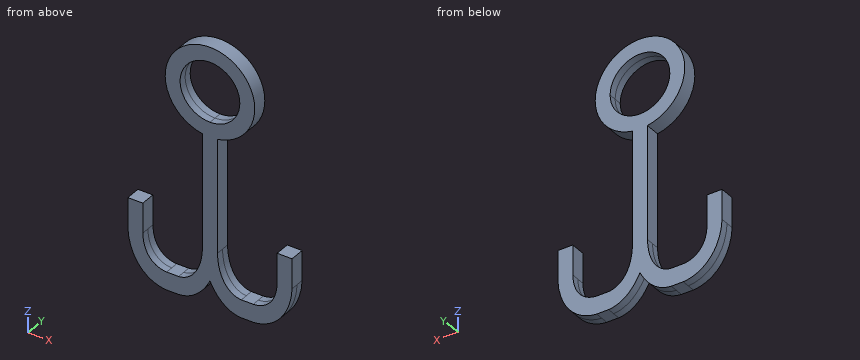
from build123d import *

# Parameters (mm, degrees)
F0_W     = 25.4
F0_H     = 38.1
F0_W_2   = 31.75
F0_H_2   = 63.5
F1_DEPTH = 15.875


with BuildPart() as f1:
    # F0 (on Front) → F1 (new body, symmetric)
    with BuildSketch(Plane.XZ):
        with BuildLine():
            Line((-15.875, -103.8391655019), (-15.875, -345.1981674205))
            Line((-15.875, -345.1981674205), (0, -345.1981674205))
            Line((0, -345.1981674205), (0, -105.1713989452))
            ThreePointArc((0, -105.1713989452), (-7.9654012916, -104.8377562407), (-15.875, -103.8391655019))
        make_face()
        with BuildLine():
            add(Edge.make_bspline(
                [(0, -409.482145582), (-10.3991862171, -388.0156164118), (-15.7271620535, -363.9765002128), (-15.875, -345.1981674205)],
                knots=[81.5477604067, 81.5477604067, 81.5477604067, 81.5477604067, 143.8364349915, 143.8364349915, 143.8364349915, 143.8364349915], degree=3))
            add(Edge.make_bspline(
                [(-66.675, -424.8878848455), (-44.6960218251, -423.8382875919), (-17.5926852971, -402.3276865482), (-15.875, -345.1981674205)],
                knots=[0, 0, 0, 0, 94.5044499655, 94.5044499655, 94.5044499655, 94.5044499655], degree=3))
            Line((-66.675, -424.8878848455), (-66.675, -462.9878848455))
            add(Edge.make_bspline(
                [(-66.675, -462.9878848455), (-35.9209941881, -461.2803468487), (-13.6145190391, -437.5859283193), (0, -409.482145582)],
                knots=[0, 0, 0, 0, 81.5477604067, 81.5477604067, 81.5477604067, 81.5477604067], degree=3))
        make_face()
        with BuildLine():
            Line((0, -345.1981674205), (-15.875, -345.1981674205))
            add(Edge.make_bspline(
                [(0, -409.482145582), (-10.3991862171, -388.0156164118), (-15.7271620535, -363.9765002128), (-15.875, -345.1981674205)],
                knots=[81.5477604067, 81.5477604067, 81.5477604067, 81.5477604067, 143.8364349915, 143.8364349915, 143.8364349915, 143.8364349915], degree=3))
            add(Edge.make_bspline(
                [(0, -409.482145582), (10.3991862171, -388.0156164118), (15.7271620535, -363.9765002128), (15.875, -345.1981674205)],
                knots=[81.5477604067, 81.5477604067, 81.5477604067, 81.5477604067, 143.8364349915, 143.8364349915, 143.8364349915, 143.8364349915], degree=3))
            Line((15.875, -345.1981674205), (0, -345.1981674205))
        make_face()
        with BuildLine():
            Line((0, -105.1713989452), (0, -345.1981674205))
            Line((0, -345.1981674205), (15.875, -345.1981674205))
            Line((15.875, -345.1981674205), (15.875, -103.8391655019))
            ThreePointArc((15.875, -103.8391655019), (7.9654012916, -104.8377562407), (0, -105.1713989452))
        make_face()
        with BuildLine():
            ThreePointArc((95.25, -9.9213989452), (-61.483610621, 62.8269902123), (-15.875, -103.8391655019))
            Line((-15.875, -103.8391655019), (-15.875, -91.1981674205))
            Line((-15.875, -91.1981674205), (0, -91.1981674205))
            Line((0, -91.1981674205), (15.875, -91.1981674205))
            Line((15.875, -91.1981674205), (15.875, -103.8391655019))
            ThreePointArc((15.875, -103.8391655019), (72.7483891574, -71.4050095662), (95.25, -9.9213989452))
        make_face()
        with BuildLine():
            ThreePointArc((63.5, -9.9213989452), (44.9012806053, -54.8226795505), (0, -73.4213989452))
            ThreePointArc((0, -73.4213989452), (-44.9012806053, 34.9798816602), (63.5, -9.9213989452))
        make_face(mode=Mode.SUBTRACT)
        with BuildLine():
            Line((-15.875, -91.1981674205), (-15.875, -103.8391655019))
            ThreePointArc((-15.875, -103.8391655019), (-7.9654012916, -104.8377562407), (0, -105.1713989452))
            Line((0, -105.1713989452), (0, -91.1981674205))
            Line((0, -91.1981674205), (-15.875, -91.1981674205))
        make_face()
        with Locations((-79.375, -443.9378848455)):
            Rectangle(F0_W, F0_H)
        with BuildLine():
            add(Edge.make_bspline(
                [(0, -409.482145582), (10.3991862171, -388.0156164118), (15.7271620535, -363.9765002128), (15.875, -345.1981674205)],
                knots=[81.5477604067, 81.5477604067, 81.5477604067, 81.5477604067, 143.8364349915, 143.8364349915, 143.8364349915, 143.8364349915], degree=3))
            add(Edge.make_bspline(
                [(66.675, -462.9878848455), (35.9209941881, -461.2803468487), (13.6145190391, -437.5859283193), (0, -409.482145582)],
                knots=[0, 0, 0, 0, 81.5477604067, 81.5477604067, 81.5477604067, 81.5477604067], degree=3))
            Line((66.675, -462.9878848455), (66.675, -424.8878848455))
            add(Edge.make_bspline(
                [(66.675, -424.8878848455), (44.6960218251, -423.8382875919), (17.5926852971, -402.3276865482), (15.875, -345.1981674205)],
                knots=[0, 0, 0, 0, 94.5044499655, 94.5044499655, 94.5044499655, 94.5044499655], degree=3))
        make_face()
        with BuildLine():
            Line((0, -91.1981674205), (0, -105.1713989452))
            ThreePointArc((0, -105.1713989452), (7.9654012916, -104.8377562407), (15.875, -103.8391655019))
            Line((15.875, -103.8391655019), (15.875, -91.1981674205))
            Line((15.875, -91.1981674205), (0, -91.1981674205))
        make_face()
        with BuildLine():
            Line((-92.075, -462.9878848455), (-92.075, -424.8878848455))
            add(Edge.make_bspline(
                [(-142.875, -361.3878848455), (-142.1477283955, -404.0485322475), (-118.0558662534, -423.8382875919), (-92.075, -424.8878848455)],
                knots=[0, 0, 0, 0, 81.3196778154, 81.3196778154, 81.3196778154, 81.3196778154], degree=3))
            Line((-142.875, -361.3878848455), (-174.625, -361.3878848455))
            add(Edge.make_bspline(
                [(-174.625, -361.3878848455), (-172.2625430346, -420.826792717), (-136.5549724221, -460.4062736034), (-92.075, -462.9878848455)],
                knots=[0, 0, 0, 0, 130.9086036134, 130.9086036134, 130.9086036134, 130.9086036134], degree=3))
        make_face()
        with Locations((79.375, -443.9378848455)):
            Rectangle(F0_W, F0_H)
        with Locations((-158.75, -329.6378848455)):
            Rectangle(F0_W_2, F0_H_2)
        with BuildLine():
            Line((92.075, -424.8878848455), (92.075, -462.9878848455))
            add(Edge.make_bspline(
                [(174.625, -361.3878848455), (172.2625430346, -420.826792717), (136.5549724221, -460.4062736034), (92.075, -462.9878848455)],
                knots=[0, 0, 0, 0, 130.9086036134, 130.9086036134, 130.9086036134, 130.9086036134], degree=3))
            Line((174.625, -361.3878848455), (142.875, -361.3878848455))
            add(Edge.make_bspline(
                [(142.875, -361.3878848455), (142.1477283955, -404.0485322475), (118.0558662534, -423.8382875919), (92.075, -424.8878848455)],
                knots=[0, 0, 0, 0, 81.3196778154, 81.3196778154, 81.3196778154, 81.3196778154], degree=3))
        make_face()
        with Locations((158.75, -329.6378848455)):
            Rectangle(F0_W_2, F0_H_2)
    extrude(amount=F1_DEPTH, both=True)


solid = f1.part
Geometry check sheet. Reference: the model listing, model coordinates, mm. Round coordinates to 2 decimals unless told otherwise and drop trailing zeros. Write each loop counter-clockwise with the first axis right and the second up, starting at its lowest first coordinate (ties: lowest second). Pieces come first, ordered by that corner, then holes. Notation, with made-up numbers: (57, 89) - (70, 89) arc R9 ccw to (70, 93) - close; hole circle Ø8 at (42, 63.25). An arc over 180 degrees is marked (long way). One line per item, written item: value.
1. Cross-section at B-B on z = -24.5. Record the boundary of the cut face in (x, y) (3 decimals), and give its area (3 significant figures).
The answers:
outline: (-94.128, -15.875) - (-61.804, -15.875) - (-61.804, 15.875) - (-94.128, 15.875) - close; (61.804, -15.875) - (94.128, -15.875) - (94.128, 15.875) - (61.804, 15.875) - close
area: 2,050 mm^2
2. Scan lines: L1, parallel to Z at x = 0, y = -3; L2, parallel to X at y = 8, z = -405; L3, parallel to Z at x = -38, y = 14. Record each from-to range of solid material in increasing order.
The answers:
L1: z = -409.48 to -73.42, 53.58 to 85.33
L2: x = -165.84 to -130, -32.87 to 32.87, 130 to 165.84
L3: z = -454.17 to -411.08, -97.26 to -60.8, 40.95 to 77.42
3. Cross-section at C-C on x = 55. Give the number of separate pieces and of enclosed holes in the cut face, and give its area (3 significant figures).
The answers:
separate pieces: 3
enclosed holes: 0
area: 4,150 mm^2
4. Depth check by flat-ended pin: pin 1 Ø16 at (y, z) = (-6.5, -203) entering from -X (3 decimals); pin 2 Ø8 at (y, z) = (9.5, -20) entering from +X; pin 3 Ø9.5 at (x, y) = (157.5, 5.5) entering from +Z. Enter the tip coordinate at first touch or a pass-through.
The answers:
pin 1: stops at x = -15.875
pin 2: stops at x = 95.06
pin 3: stops at z = -297.89
5. Cross-section at A-A on z = -313. Record the boundary of the cut face in (x, y) (3 decimals).
The answers:
outline: (-174.625, -15.875) - (-142.875, -15.875) - (-142.875, 15.875) - (-174.625, 15.875) - close; (-15.875, -15.875) - (15.875, -15.875) - (15.875, 15.875) - (-15.875, 15.875) - close; (142.875, -15.875) - (174.625, -15.875) - (174.625, 15.875) - (142.875, 15.875) - close
